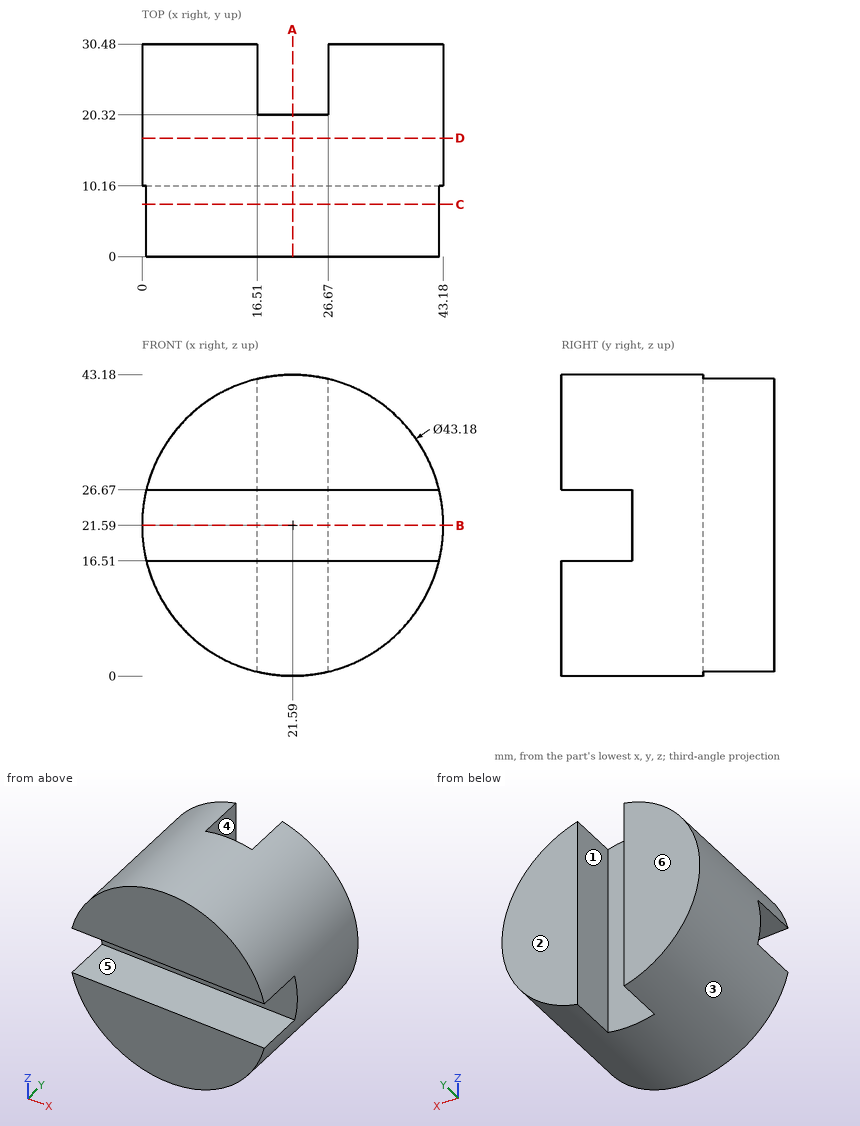
Design review of the part shown in the three views and the two pictorial views. Dimensions are in mm from the part's minimum x, y and z. A direction names the side the tool comes from. Coordinates: 2 decimals unless noted, no trailing zeros. Order: outer loops, then holes, each group sorted by start corner. A loop starts at its lowest first (then second) coordinate and runs counter-clockwise, first axis right, second up.
1) Take a section at C-C, the plane y = 7.5. Give the boundary of the cut face in (x, z), and give its area (3 significant figures).
2) Take a section at D-D, the plane y = 17. Give the boundary of the cut face in (x, z).
3) Take a section at A-A, the plane x = 21.59. Give the boundary of the cut face in (y, z).
4) Take a section at B-B, the plane z = 21.59. Give the boundary of the cut face in (x, y), and give its area (3 significant figures).
5) Mouldability with a two-part tool opening along X and no side actions: class the marked faces 1, 2 and 3 as +X half, -X half, draft (parallel to the pull), parting line (faces both ways), or undercut.
6) Wall thickness on line 1 along Y through (x, z) = (12.5, 21); line 2 along Z through (x, y) = (28.5, 8.5); line 3 along X through (y, z) = (21, 20.5): over which ranges is each line inside the solid? List them lowest first.
7) For the marked faces 4, 5 and 6, list the 3-axis set-ups (+Z, -Z, +X, -X, +Y, -Y) from which the entire face can be reached by the end or side of a thin tool; tool diameter is ignored.
8) Clearance check with flat-ended pins moving along their axes: pin 1 (11 mm diameter, centred on x = 28.5, y = 6.5, fed in from -Z); pin 2 (1.5 mm diameter, centred on y = 15, z = 29.5, fed in from +X); pin 3 (5 mm diameter, centred on y = 23.5, z = 29, fed in from +X). State where each tip first meets the part, or that it passes through.
Returned:
1. outline: (0.61, 16.51) arc R21.59 ccw to (42.57, 16.51) - close; (0.61, 26.67) - (42.57, 26.67) arc R21.59 ccw to start
1. area: 1,030 mm2
2. outline: circle Ø43.18 at (21.59, 21.59)
3. outline: (0, 0) - (20.32, 0) - (20.32, 43.18) - (0, 43.18) - (0, 26.67) - (10.16, 26.67) - (10.16, 16.51) - (0, 16.51) - close
4. outline: (0, 10.16) - (43.18, 10.16) - (43.18, 30.48) - (26.67, 30.48) - (26.67, 20.32) - (16.51, 20.32) - (16.51, 30.48) - (0, 30.48) - close
4. area: 774 mm2
5. face 1: undercut
5. face 2: draft
5. face 3: parting line
6. line 1: y = 10.16 to 30.48
6. line 2: z = 1.14 to 16.51, 26.67 to 42.04
6. line 3: x = 0.03 to 16.51, 26.67 to 43.15
7. face 4: +Z, -Z, +Y
7. face 5: +X, -X, -Y
7. face 6: +Z, -Z, +X, -X, +Y
8. pin 1: stops at z = 0.05
8. pin 2: stops at x = 41.96
8. pin 3: stops at x = 42.61
